Source: CAD feature listing. Evaluate the final solid. Frame: model axes, mm. A direction names the side the tool comes from. Give positions to 0.01 mm unless a question says otherwise; leave off trailing zeros. Loops run counter-clockwise (first coordinate to the right, second up) from the corner with the lowest first, then second, coordinate; pieces in that order, holes last.
Autodesk Inventor part; units mm, degrees
ref_plane "YZ Plane" through (0, 0, 0) normal (1, 0, 0) x (0, 1, 0)
ref_plane "XZ Plane" through (0, 0, 0) normal (0, 1, 0) x (-1, 0, 0)
ref_plane "XY Plane" through (0, 0, 0) normal (0, 0, 1) x (1, 0, 0)
sketch "Sketch1" plane through (0, 0, 0) normal (0, 1, 0) x (-1, 0, 0)
  line L0 (0, 0) -> (72, 0)
  line L1 (72, 0) -> (72, -90)
  line L2 (72, -90) -> (0, -90)
  line L3 (0, -90) -> (0, 0)
  dimension "d0" = 72
  dimension "d1" = 90
extrude "Extrusion1" add sketch "Sketch1" along normal blind 5
sketch "Sketch2" plane through (0, 0, 0) normal (0, -1, 0) x (1, 0, 0)
  line L0 (-72, 0) -> (-72, -90)
  line L1 (-72, -90) -> (0, -90)
  circle A0 centre (-36, -72) radius 8.75
  circle A1 centre (-36, -18) radius 8.75
  circle A2 centre (-36, -18) radius 11.5
  circle A3 centre (-36, -72) radius 11.5
  dimension "d4" = 17.5
  dimension "d5" = 23
  dimension "d6" = 54
  dimension "d7" = 18
  dimension "d8" = 36
extrude "Extrusion2" add sketch "Sketch2" along normal blind 10.7
sketch "Sketch3" plane through (-36, 0, -18) normal (0, -1, 0) x (1, 0, 0)
  circle A0 centre (0, 0) radius 8.75
  circle A1 centre (0, -54) radius 8.75
  point P0 (36, 18)
extrude "Extrusion3" cut sketch "Sketch3" against normal up to surface (5 mm away)
sketch "Sketch4" plane through (0, 0, 0) normal (0, -1, 0) x (1, 0, 0)
  line L0 (0, 0) -> (-72, 0)
  line L1 (-72, 0) -> (-72, -90)
  line L2 (0, -90) -> (0, 0)
  circle A0 centre (-21, -45) radius 13
  circle A1 centre (-51, -45) radius 13
  dimension "d14" = 26
  dimension "d16" = 21
  dimension "d17" = 21
  dimension "d18" = 45
extrude "Extrusion4" cut sketch "Sketch4" against normal up to surface (5 mm away)
sketch "Sketch5" plane through (0, 0, 0) normal (0, -1, 0) x (1, 0, 0)
  circle A0 centre (-21, -45) radius 13
  circle A1 centre (-51, -45) radius 13
  circle A2 centre (-9, -57) radius 1.5
  circle A3 centre (-9, -33) radius 1.5
  circle A4 centre (-33, -57) radius 1.5
  circle A5 centre (-33, -33) radius 1.5
  circle A6 centre (-39, -33) radius 1.5
  circle A7 centre (-39, -57) radius 1.5
  circle A8 centre (-63, -57) radius 1.5
  circle A9 centre (-63, -33) radius 1.5
  dimension "d21" = 3
  dimension "d22" = 24
  dimension "d23" = 24
  dimension "d24" = 24
  dimension "d25" = 12
  dimension "d26" = 12
  dimension "d27" = 12
extrude "Extrusion5" cut sketch "Sketch5" against normal up to surface (5 mm away) contours A2 | A3 | A4 | A5 | A6 | A7 | A8 | A9
sketch "Sketch6" plane through (0, 5, 0) normal (0, 1, 0) x (1, 0, 0)
  circle A0 centre (-39, 57) radius 1.5
  circle A1 centre (-33, 33) radius 1.5
  circle A2 centre (-33, 57) radius 1.5
  circle A3 centre (-39, 33) radius 1.5
  line L0 (-39, 60.1754) -> (-36.25, 58.5877)
  line L1 (-36.25, 58.5877) -> (-36.25, 55.4123)
  line L2 (-36.25, 55.4123) -> (-39, 53.8246)
  line L3 (-39, 53.8246) -> (-41.75, 55.4123)
  line L4 (-41.75, 55.4123) -> (-41.75, 58.5877)
  line L5 (-41.75, 58.5877) -> (-39, 60.1754)
  line L6 (-39, 36.1754) -> (-36.25, 34.5877)
  line L7 (-36.25, 34.5877) -> (-36.25, 31.4123)
  line L8 (-36.25, 31.4123) -> (-39, 29.8246)
  line L9 (-39, 29.8246) -> (-41.75, 31.4123)
  line L10 (-41.75, 31.4123) -> (-41.75, 34.5877)
  line L11 (-41.75, 34.5877) -> (-39, 36.1754)
  line L12 (-33, 36.1754) -> (-30.25, 34.5877)
  line L13 (-30.25, 34.5877) -> (-30.25, 31.4123)
  line L14 (-30.25, 31.4123) -> (-33, 29.8246)
  line L15 (-33, 29.8246) -> (-35.75, 31.4123)
  line L16 (-35.75, 31.4123) -> (-35.75, 34.5877)
  line L17 (-35.75, 34.5877) -> (-33, 36.1754)
  line L18 (-33, 60.1754) -> (-30.25, 58.5877)
  line L19 (-30.25, 58.5877) -> (-30.25, 55.4123)
  line L20 (-30.25, 55.4123) -> (-33, 53.8246)
  line L21 (-33, 53.8246) -> (-35.75, 55.4123)
  line L22 (-35.75, 55.4123) -> (-35.75, 58.5877)
  line L23 (-35.75, 58.5877) -> (-33, 60.1754)
  dimension "d30" = 5.5
extrude "Extrusion6" cut sketch "Sketch6" against normal blind 2.5
properties part number "XCarriageV9Top" material "ABS Plastic"
1) Cut plane D-D (y = -8.5). Return loops of the section in (x, z), and give its area (3 significant figures).
Checks:
outline: circle Ø23 at (-36, -72); circle Ø23 at (-36, -18); hole circle Ø17.5 at (-36, -72); hole circle Ø17.5 at (-36, -18)
area: 350 mm2
2) Pull-direction query (Z, two-part tool) for faces 4 (the flat face through (-35, 2, 0)), 5 (the flat face through (0, 2, -46)), 6 (the cylindrical face through (-60.58, 2.46, -36.21)), 7 (the flat face through (-40.36, 3.77, -30.61)); classes: released by +Z, released by -Z, zero draft, split by the parting line, or undercut.
Checks:
face 4: released by +Z
face 5: zero draft
face 6: undercut
face 7: undercut
3) Cut plane A-A (z = -45). Return loops of the section in (x, y), and give its area (3 significant figures).
Checks:
outline: (-72, 0) - (-64, 0) - (-64, 5) - (-72, 5) - close; (-38, 0) - (-34, 0) - (-34, 5) - (-38, 5) - close; (-8, 0) - (0, 0) - (0, 5) - (-8, 5) - close
area: 100 mm2
4) Cut plane B-B (x = -63). Return loops of the section in (y, z).
Checks:
outline: (0, -90) - (5, -90) - (5, -58.5) - (0, -58.5) - close; (0, -55.5) - (5, -55.5) - (5, -50) - (0, -50) - close; (0, -40) - (5, -40) - (5, -34.5) - (0, -34.5) - close; (0, -31.5) - (5, -31.5) - (5, 0) - (0, 0) - close
5) Ray query, probe 1 along Z at (x, y) = (-42, -6.75); probe 2 along Z at (x, y) = (-39, 0.7); probe 3 along Z at (x, y) = (-9, 3.55). Return the intervals inside material, ascending.
Checks:
probe 1: z = -81.81 to -78.37, -65.63 to -62.19, -27.81 to -24.37, -11.63 to -8.19
probe 2: z = -90 to -80.22, -63.78 to -58.5, -55.5 to -50, -40 to -34.5, -31.5 to -26.22, -9.78 to 0
probe 3: z = -90 to -58.5, -55.5 to -50, -40 to -34.5, -31.5 to 0
6) Reachability of faces 1 (the flat face through (-35, 0, -44)), 2 (the cylindrical face through (-27.654, -2.96, -15.372)), 3 (the flat face through (-37.606, 3.768, -54.63)) from +Z, -Z, +X, -X, +Y, -Y: full face, straight path, thin tool, end or side. Return the list, or none.
Checks:
face 1: -Y
face 2: +Y, -Y
face 3: +Y
7) Cut plane C-C (x = -21). Return loops of the section in (y, z).
Checks:
outline: (0, -90) - (5, -90) - (5, -58) - (0, -58) - close; (0, -32) - (5, -32) - (5, 0) - (0, 0) - close
8) Contact query for flat-ended pins moving along their axis: P1, Ø5, axis at y = 0, z = -70.5, coming from the +X side; P2, Ø4, axis at x = -9, z = -33, coming from the -Y side; P3, Ø6, axis at x = -39, y = -6, coming from the -Z side. Output: stop coordinate, or through.
Checks:
P1: stops at x = 0
P2: stops at y = 0
P3: stops at z = -83.5
